Verification items for the finished model (mm, model axes). A direction names the side the tool comes from. Coordinates: 2 decimals unless noted, no trailing zeros. Write each loop counter-clockwise with the first axis right and the second up, starting at its lowest first coordinate (ties: lowest second). Pieces come first, ordered by that corner, then holes. Notation, with made-up numbers: (66.25, 58.25) -> (78.25, 58.25) arc R17 ccw to (78.25, 71.25) -> close; hole circle Ø11 at (4.5, 52.5). An arc over 180 degrees is marked (long way). Answer in a Markdown table with one row per item.
Autodesk Inventor part; units mm, degrees
ref_plane "YZ Plane" through (0, 0, 0) normal (1, 0, 0) x (0, 1, 0)
ref_plane "XZ Plane" through (0, 0, 0) normal (0, 1, 0) x (-1, 0, 0)
ref_plane "XY Plane" through (0, 0, 0) normal (0, 0, 1) x (1, 0, 0)
sketch "Sketch1" plane through (0, 0, 0) normal (0, 0, 1) x (1, 0, 0)
  line L0 (0, 0) -> (2.5, 0) construction
  line L1 (2.5, 4.5) -> (2.5, -4.5)
  line L2 (2.5, -4.5) -> (9, -4.5)
  line L3 (9, -4.5) -> (9, -3.25)
  line L4 (9, -3.25) -> (6.05, -3.25)
  line L5 (6.05, -3.25) -> (6.05, 3.25)
  line L6 (6.05, 3.25) -> (9, 3.25)
  line L7 (9, 3.25) -> (9, 4.5)
  line L8 (9, 4.5) -> (2.5, 4.5)
  line L9 (0, -6.3) -> (0, 6.3)
  dimension "d0" = 2.5
  dimension "d1" = 6.5
  dimension "d2" = 9
  dimension "d3" = 9
  dimension "d4" = 6.05
revolve "Revolution1" add sketch "Sketch1" angle 360 about axis through (0, -10, 0) along (0, 1, 0)
sketch "Sketch2" plane through (0, 4.5, 0) normal (0, 1, 0) x (1, 0, 0)
  circle A0 centre (0, 0) radius 4.5
  dimension "d6" = 9
extrude "Extrusion1" cut sketch "Sketch2" against normal blind 3
mirror "Mirror1" about plane through (0, 0, 0) normal (0, 1, 0) of "Extrusion1"
properties part number "Idler Pulley" material "Aluminum 6061"
1. Release check for a two-part mould opening along X. For faces 1 (the face through (5.589, 0.046, 2.317)), 2 (the face through (-2, -1.5, 2)), 3 (the face through (2, 3.25, 6)) record: released by +X, released by -X, zero draft, split by the parting line, or undercut.
Findings below:
| item | result |
|---|---|
| face 1 | split by the parting line |
| face 2 | undercut |
| face 3 | zero draft |
2. Sectioned sample at D-D, the plane z = -7.25. Record the cut outline in (x, y).
Findings below:
| item | result |
|---|---|
| outline | (-5.33, -4.5) -> (5.33, -4.5) -> (5.33, -3.25) -> (-5.33, -3.25) -> close; (-5.33, 3.25) -> (5.33, 3.25) -> (5.33, 4.5) -> (-5.33, 4.5) -> close |
3. Go/stop test with flat-tipped pins: pin 1 (5.5 mm diameter, centred on x = 0, z = 0, fed in from -Y); pin 2 (1 mm diameter, centred on y = 3.5, z = -3.5, fed in from -X); pin 3 (8 mm diameter, centred on x = 0, z = 0, fed in from +Y). Record where each tip stops, or that it passes through.
Findings below:
| item | result |
|---|---|
| pin 1 | stops at y = -1.5 |
| pin 2 | stops at x = -8.49 |
| pin 3 | stops at y = 1.5 |
4. Sectioned sample at C-C, the plane y = -3.5. Record the cut outline in (x, z), and give its area (3 significant figures).
Findings below:
| item | result |
|---|---|
| outline | circle Ø18 at (0, 0); hole circle Ø9 at (0, 0) |
| area | 191 mm² |
5. Access from +Z, -Z, +X, -X, +Y, -Y to the whole of each face (thin tool, end or side, straight path). Record for faces 4 (the face through (-0.59, -3.02, 4.46)), 5 (the face through (-0.59, 3.02, -4.46)), 6 (the face through (4, 4.5, 4)), 7 (the face through (2, -3.25, 6)).
Findings below:
| item | result |
|---|---|
| face 4 | -Y |
| face 5 | +Y |
| face 6 | +Z, -Z, +X, -X, +Y |
| face 7 | none |
6. Material ranges on probe 1 along Z at (x, y) = (0, -0.4); probe 2 along Z at (x, y) = (0, -2.9); probe 3 along Y at (x, z) = (-5.25, 7), recorded low to high. Write a range as from..to.
Findings below:
| item | result |
|---|---|
| probe 1 | z = -6.05..-2.5, 2.5..6.05 |
| probe 2 | z = -6.05..-4.5, 4.5..6.05 |
| probe 3 | y = -4.5..-3.25, 3.25..4.5 |
7. Sectioned sample at A-A, the plane x = 0. Record the cut outline in (y, z), and give its area (4 significant figures).
Findings below:
| item | result |
|---|---|
| outline | (-4.5, -9) -> (-3.25, -9) -> (-3.25, -6.05) -> (3.25, -6.05) -> (3.25, -9) -> (4.5, -9) -> (4.5, -4.5) -> (1.5, -4.5) -> (1.5, -2.5) -> (-1.5, -2.5) -> (-1.5, -4.5) -> (-4.5, -4.5) -> close; (-4.5, 4.5) -> (-1.5, 4.5) -> (-1.5, 2.5) -> (1.5, 2.5) -> (1.5, 4.5) -> (4.5, 4.5) -> (4.5, 9) -> (3.25, 9) -> (3.25, 6.05) -> (-3.25, 6.05) -> (-3.25, 9) -> (-4.5, 9) -> close |
| area | 54.65 mm² |
8. Sectioned sample at B-B, the plane z = 0. Record the cut outline in (x, y), and give its area (4 significant figures).
Findings below:
| item | result |
|---|---|
| outline | (-9, -4.5) -> (-4.5, -4.5) -> (-4.5, -1.5) -> (-2.5, -1.5) -> (-2.5, 1.5) -> (-4.5, 1.5) -> (-4.5, 4.5) -> (-9, 4.5) -> (-9, 3.25) -> (-6.05, 3.25) -> (-6.05, -3.25) -> (-9, -3.25) -> close; (2.5, -1.5) -> (4.5, -1.5) -> (4.5, -4.5) -> (9, -4.5) -> (9, -3.25) -> (6.05, -3.25) -> (6.05, 3.25) -> (9, 3.25) -> (9, 4.5) -> (4.5, 4.5) -> (4.5, 1.5) -> (2.5, 1.5) -> close |
| area | 54.65 mm² |
